```python
from build123d import *

# Parameters (mm, degrees)
SKETCH1_R           = 8.5
BOSS_EXTRUDE1_DEPTH = 4
BOSS_EXTRUDE2_DEPTH = 13
SKETCH3_W           = 2.2
SKETCH3_H           = 6.3
CUT_EXTRUDE1_DEPTH  = 3.5
SKETCH4_R           = 1.75
CUT_EXTRUDE2_DEPTH  = 47.663174732
SKETCH6_W           = 13.5
SKETCH6_H           = 2
CUT_EXTRUDE4_DEPTH  = 47.663174732
SKETCH7_W           = 2
SKETCH7_H           = 25
BOSS_EXTRUDE3_DEPTH = 17
CUT_EXTRUDE5_DEPTH  = 72
SKETCH9_R           = 1.75
BOSS_EXTRUDE4_DEPTH = 6
SKETCH10_R          = 2.85
CUT_EXTRUDE6_DEPTH  = 8


with BuildPart() as part:
    # Sketch1 → Boss-Extrude1 (new body)
    with BuildSketch(Plane.XY):
        Polygon((-10.41954023, 18.706896552), (-10.41954023, -6.293103448), (38.58045977, -6.293103448), (38.58045977, 18.706896552), (19.08045977, 18.706896552), (19.08045977, 15.706896552), (14.08045977, 15.706896552), (9.08045977, 15.706896552), (9.08045977, 18.706896552), align=None)
        with BuildLine():
            ThreePointArc((10.46545977, -0.583103448), (8.61545977, 1.266896552), (10.46545977, 3.116896552))
            Line((10.46545977, 3.116896552), (17.69545977, 3.116896552))
            ThreePointArc((17.69545977, 3.116896552), (19.54545977, 1.266896552), (17.69545977, -0.583103448))
            Line((17.69545977, -0.583103448), (10.46545977, -0.583103448))
        make_face(mode=Mode.SUBTRACT)
        with Locations((1.08045977, 8.706896552)):
            Circle(SKETCH1_R, mode=Mode.SUBTRACT)
        with Locations((27.08045977, 8.706896552)):
            Circle(SKETCH1_R, mode=Mode.SUBTRACT)
    extrude(amount=BOSS_EXTRUDE1_DEPTH)

    # Sketch2 → Boss-Extrude2 (add)
    with BuildSketch(Plane.XY.offset(4)):
        Polygon((14.08045977, -1.293103448), (38.58045977, -1.293103448), (38.58045977, -6.293103448), (-10.41954023, -6.293103448), (-10.41954023, -1.293103448), align=None)
    extrude(amount=BOSS_EXTRUDE2_DEPTH)

    # Sketch3 → Cut-Extrude1 (cut)
    with BuildSketch(Plane(origin=(0, -1.293103448, 0), x_dir=(1, 0, 0), z_dir=(0, 1, 0))):
        with Locations((10.08045977, -9.65)):
            Rectangle(SKETCH3_W, SKETCH3_H)
        with Locations((18.08045977, -9.65)):
            Rectangle(SKETCH3_W, SKETCH3_H)
    extrude(amount=-CUT_EXTRUDE1_DEPTH, mode=Mode.SUBTRACT)

    # Sketch4 → Cut-Extrude2 (cut, through all)
    with BuildSketch(Plane(origin=(0, -1.293103448, 0), x_dir=(1, 0, 0), z_dir=(0, 1, 0))):
        with Locations(Location((14.08045977, -9.15, 0), (0, 0, 270))):
            Circle(SKETCH4_R)
        with Locations(Location((33.58045977, -12, 0), (0, 0, 270))):
            Circle(SKETCH4_R)
        with Locations(Location((-5.41954023, -12, 0), (0, 0, 90))):
            Circle(SKETCH4_R)
    extrude(amount=-CUT_EXTRUDE2_DEPTH, mode=Mode.SUBTRACT)

    # Sketch6 → Cut-Extrude4 (cut, through all)
    with BuildSketch(Plane(origin=(0, -1.293103448, 0), x_dir=(1, 0, 0), z_dir=(0, 1, 0))):
        with Locations((7.33045977, -16)):
            Rectangle(SKETCH6_W, SKETCH6_H)
        with Locations((20.83045977, -16)):
            Rectangle(SKETCH6_W, SKETCH6_H)
    extrude(amount=-CUT_EXTRUDE4_DEPTH, mode=Mode.SUBTRACT)

    # Sketch7 → Boss-Extrude3 (add)
    with BuildSketch(Plane(origin=(0, 0, 0), x_dir=(-1, 0, 0), z_dir=(0, 0, -1))):
        with Locations((-39.58045977, 6.206896552)):
            Rectangle(SKETCH7_W, SKETCH7_H)
        with Locations((11.41954023, 6.206896552)):
            Rectangle(SKETCH7_W, SKETCH7_H)
    extrude(amount=-BOSS_EXTRUDE3_DEPTH)

    # Sketch8 → Cut-Extrude5 (cut)
    with BuildSketch(Plane(origin=(40.58045977, 0, 0), x_dir=(0, 0, -1), z_dir=(1, 0, 0))):
        Polygon((-4, 18.706896552), (-17, -1.293103448), (-17, 18.706896552), align=None)
    extrude(amount=-CUT_EXTRUDE5_DEPTH, mode=Mode.SUBTRACT)

    # Sketch9 → Boss-Extrude4 (add)
    with BuildSketch(Plane(origin=(0, -6.293103448, 0), x_dir=(-1, 0, 0), z_dir=(0, -1, 0))):
        Polygon((-40.58045977, 0), (-40.58045977, -17), (-27.58045977, -17), (-27.58045977, -15), (-0.58045977, -15), (-0.58045977, -17), (12.41954023, -17), (12.41954023, 0), align=None)
        with Locations(Location((5.41954023, -12, 0), (0, 0, 90))):
            Circle(SKETCH9_R, mode=Mode.SUBTRACT)
        with Locations(Location((-14.08045977, -9.15, 0), (0, 0, 270))):
            Circle(SKETCH9_R, mode=Mode.SUBTRACT)
        with Locations(Location((-33.58045977, -12, 0), (0, 0, 270))):
            Circle(SKETCH9_R, mode=Mode.SUBTRACT)
    extrude(amount=BOSS_EXTRUDE4_DEPTH)

    # Sketch10 → Cut-Extrude6 (cut)
    with BuildSketch(Plane(origin=(0, -12.293103448, 0), x_dir=(-1, 0, 0), z_dir=(0, -1, 0))):
        with Locations(Location((-14.08045977, -9.15, 0), (0, 0, 90))):
            Circle(SKETCH10_R)
    extrude(amount=-CUT_EXTRUDE6_DEPTH, mode=Mode.SUBTRACT)


solid = part.part
```
Input: part model. Units: mm. Frame: model coordinates. A direction names the side the tool comes from. Give positions to 0.01 mm unless a question says otherwise; leave off trailing zeros. Order: outer loops, then holes, each group sorted by start corner. A loop starts at its lowest first (then second) coordinate and runs counter-clockwise, first axis right, second up. Notation, with made-up numbers: (-19.5, 50) - (36.5, 50) arc R16 cw to (36.5, 63) - close; hole circle Ø9 at (-36.75, 88.25). An arc over 180 degrees is marked (long way). One line per item, written item: value.
1. Cut plane D-D, the plane y = 14. Output: boundary loops of the cut face in (x, z).
Determined:
outline: (-12.42, 0) - (-5.57, 0) - (-5.57, 4) - (-10.42, 4) - (-10.42, 7.06) - (-12.42, 7.06) - close; (7.73, 0) - (20.43, 0) - (20.43, 4) - (7.73, 4) - close; (33.73, 0) - (40.58, 0) - (40.58, 7.06) - (38.58, 7.06) - (38.58, 4) - (33.73, 4) - close
2. Reachability of faces 1 (the face through (19.18, -3, 10)), 2 (the face through (14, -1.293, 12)), 3 (the face through (0.58, -7, 16)), 4 (the face through (14, -0.583, 2)) from +Z, -Z, +X, -X, +Y, -Y: full face, straight path, thin tool, end or side. Return the list, or none.
Determined:
face 1: +Y
face 2: +Z, +Y
face 3: +Z, +Y, -Y
face 4: +Z, -Z
3. Cut plane B-B, the plane z = 9.15. Output: boundary loops of the cut face in (x, y), and give its area (3 significant figures).
Determined:
outline: (-12.42, -12.29) - (11.23, -12.29) - (11.23, -4.29) - (12.33, -4.29) - (12.33, -1.29) - (11.18, -1.29) - (11.18, -4.79) - (8.98, -4.79) - (8.98, -1.29) - (-10.42, -1.29) - (-10.42, 10.78) - (-12.42, 10.78) - close; (15.83, -4.29) - (16.93, -4.29) - (16.93, -12.29) - (40.58, -12.29) - (40.58, 10.78) - (38.58, 10.78) - (38.58, -1.29) - (19.18, -1.29) - (19.18, -4.79) - (16.98, -4.79) - (16.98, -1.29) - (15.83, -1.29) - close
area: 560 mm2
4. Cut plane A-A, the plane x = 21. Output: boundary loops of the cut face in (y, z).
Determined:
outline: (-12.29, 0) - (2.77, 0) - (2.77, 4) - (-1.29, 4) - (-1.29, 15) - (-12.29, 15) - close; (14.65, 0) - (18.71, 0) - (18.71, 4) - (14.65, 4) - close
5. Draft query along X for faces 5 (the face through (-12.42, 0, 7)), 6 (the face through (10, -3, 6.5)), 7 (the face through (14, -12.293, 5)). Return one class per face: released by +X, released by -X, zero draft, split by the parting line, or undercut.
Determined:
face 5: released by -X
face 6: undercut
face 7: zero draft
6. Cut plane C-C, the plane y = -9.5. Output: boundary loops of the cut face in (x, z), and give its area (3 significant figures).
Determined:
outline: (-12.42, 0) - (40.58, 0) - (40.58, 17) - (27.58, 17) - (27.58, 15) - (0.58, 15) - (0.58, 17) - (-12.42, 17) - close; hole circle Ø3.5 at (-5.42, 12); hole circle Ø5.7 at (14.08, 9.15); hole circle Ø3.5 at (33.58, 12)
area: 802 mm2
7. Pin query (flat end, axial travel): pin 1 Ø5 at (y, z) = (5.5, 15) entering from -X; pin 2 Ø3 at (x, z) = (13, 2) entering from +Y; pin 3 Ø10 at (x, y) = (20.5, 7) entering from +Z; pin 4 Ø1.1 at (x, z) = (18, 10.5) entering from +Y. Return the tip coordinate at first contact, or that it passes through.
Determined:
pin 1: x = -12.42
pin 2: y = 15.71
pin 3: z = 4
pin 4: y = -4.79
8. Line query: probe 1 along X at (y, z) = (-3.5, 9.15); probe 2 along X at (y, z) = (8.5, 0.5); probe 3 along X at (y, z) = (4.5, 5). Output: solid intervals per line, ascending.
Determined:
probe 1: -12.42 to 8.98, 11.18 to 12.33, 15.83 to 16.98, 19.18 to 40.58
probe 2: -12.42 to -7.42, 9.58 to 18.58, 35.58 to 40.58
probe 3: -12.42 to -10.42, 38.58 to 40.58
